Could you check a few things on this model? Use its own coordinates, in mm. A direction names the side the tool comes from. Give positions to 0.01 mm unless a question says otherwise; leave off trailing zeros. Loops run counter-clockwise (first coordinate to the right, second up) from the corner with the lowest first, then second, coordinate; pieces in that order, holes last. Notation, with made-up numbers: M -24.5,72 L 0.5,72 A19 cw 0.5,85 Z; hole C 38,47 d3. An arc over 180 degrees is marked long. Use CSV: the item, a comma, the result in double quotes.
```python
from build123d import *

# Parameters (mm, degrees)
F0_W     = 24
F0_H     = 28.575
F1_DEPTH = 54.991
F2_T     = -2.54
F3_W     = 18.5978077352
F3_H     = 17.8960040212
F4_DEPTH = 76.2
F5_W     = 36.7379160598
F5_H     = 28.575
F6_DEPTH = 12.7
F7_W     = 20.9140316583
F7_H     = 11.9311325252
F8_DEPTH = 25.4


# Not quite as in the source:
# - a feature of the source that left no trace in its solid (it failed there, or was rolled back) is left out


with BuildPart() as f1:
    # F0 (on Front) → F1 (new body, symmetric)
    with BuildSketch(Plane.XZ):
        Polygon((-76.2, -28.575), (76.2, -28.575), (76.2, 28.575), (0, 28.575), (28.2, 0), (-52.2, 0), (-76.2, 0), align=None)
        Polygon((-104.4, 28.575), (-76.2, 0), (-76.2, 28.575), align=None)
        with Locations((-64.2, 14.2875)):
            Rectangle(F0_W, F0_H)
        Polygon((28.2, 0), (0, 28.575), (-52.2, 28.575), (-52.2, 0), align=None)
    extrude(amount=F1_DEPTH, both=True)

    # F2
    f2_openings = [f1.faces().sort_by_distance(p)[0] for p in [
        (-3.78476, -54.991, 0.842286),
    ]]
    offset(amount=F2_T, openings=f2_openings, kind=Kind.INTERSECTION)

    # F3 (on Right) → F4 (join, through all)
    with BuildSketch(Plane.YZ):
        with Locations((25.7912892848, 3.5090195015)):
            Rectangle(F3_W, F3_H)
    extrude(amount=-F4_DEPTH)

    # F5 (on face) → F6 (join)
    with BuildSketch(Plane.YZ.offset(76.2)):
        with Locations((4.6260296367, -14.2875)):
            Rectangle(F5_W, F5_H)
    extrude(amount=F6_DEPTH)

    # F7 (on face) → F8 (cut)
    with BuildSketch(Plane.YZ.offset(76.2)):
        with Locations((-15.9690368455, 7.5058937073)):
            Rectangle(F7_W, F7_H)
    extrude(amount=-F8_DEPTH, mode=Mode.SUBTRACT)


solid = f1.part
```
1. Which directions (+Z, -Z, +X, -X, +Y, -Y) give clear straight access to the entire face, cutting with the end or side of a thin tool? Please do faces 5 (the face through (82, 22.995, -14)), 6 (the face through (-38, 16.492, 3)), 7 (the face through (-38, 35.09, 3)).
Outcome:
face 5,"+Z, -Z, +X, +Y"
face 6,"-Y"
face 7,"none"
2. I'm going to push flat-ended pins straight in: pin 1 Ø10 at (x, z) = (82.5, -20) entering from +Y (3 decimals); pin 2 Ø4.5 at (y, z) = (24.5, 9.5) entering from -X; pin 3 Ø1 at (y, z) = (-5.5, -14.5) entering from -X. Where does each tip first touch, or does it pass through?
Outcome:
pin 1,"y = 22.995"
pin 2,"x = -87.8"
pin 3,"x = -76.2"
3. I want a section at B-B, the plane z = 6. List the corners of the cut face in (x, y) for me, then the cut area to 3 significant figures.
Outcome:
outline,"M -82.12,-54.99 L -78.55,-54.99 L -78.55,52.45 L 73.66,52.45 L 73.66,-5.51 L 76.2,-5.51 L 76.2,54.99 L -82.12,54.99 Z; M -76.2,16.49 L 0,16.49 L 0,35.09 L -76.2,35.09 Z; M 73.66,-54.99 L 76.2,-54.99 L 76.2,-26.43 L 73.66,-26.43 Z"
area,"2,420 mm2"
4. If we mould it in two halves opening along X, with no side actions, what happens to faces 1 (the face through (-86.165, -2.022, 13.714)), 2 (the face through (88.9, 4, -14)), 3 (the face through (82, 4, 0)), 4 (the face through (-76.2, 26, 8))? For each: +X half, -X half, draft (parallel to the pull), parting line (faces both ways), or undercut.
Outcome:
face 1,"undercut"
face 2,"+X half"
face 3,"draft"
face 4,"undercut"
5. I want a section at D-D, the plane z = -3. List the corners of the cut face in (x, y) for me.
Outcome:
outline,"M -76.2,-54.99 L -73.66,-54.99 L -73.66,16.49 L 0,16.49 L 0,35.09 L -73.66,35.09 L -73.66,52.45 L 73.66,52.45 L 73.66,-54.99 L 76.2,-54.99 L 76.2,-13.74 L 88.9,-13.74 L 88.9,22.99 L 76.2,22.99 L 76.2,54.99 L -76.2,54.99 Z"
6. I want a section at A-A, the plane y = 10.5. List the corners of the cut face in (x, z) for me (3 decimals), then the cut area to 3 significant figures.
Outcome:
outline,"M -104.4,28.575 L -76.2,0 L -76.2,-28.575 L 88.9,-28.575 L 88.9,0 L 76.2,0 L 76.2,28.575 Z; hole M -98.325,26.035 L -73.66,1.042 L -73.66,-26.035 L 73.66,-26.035 L 73.66,26.035 Z"
area,"1,500 mm2"
7. I want a section at C-C, the plane x = 7. List the corners of the cut face in (y, z) for me (3 decimals).
Outcome:
outline,"M -54.991,-28.575 L 54.991,-28.575 L 54.991,28.575 L -54.991,28.575 L -54.991,26.035 L 52.451,26.035 L 52.451,-26.035 L -54.991,-26.035 Z"
8. Please list where these lines run through material, in increasing order: line 1 (X direction, y = -21, z = -16.5); line 2 (Z direction, x = -32, y = 13) (3 decimals); line 3 (Y direction, x = -46, z = 5).
Outcome:
line 1,"-76.2 to -73.66, 73.66 to 76.2"
line 2,"-28.575 to -26.035, 26.035 to 28.575"
line 3,"16.49 to 35.09, 52.45 to 54.99"
